```python
from build123d import *

# Parameters (mm, degrees)
BOSS_EXTRUDE1_DEPTH = 8
SKETCH4_R           = 2.6
CUT_EXTRUDE1_DEPTH  = 23
SKETCH5_R           = 1.5
CUT_EXTRUDE2_DEPTH  = 19.692452066


with BuildPart() as part:
    # Sketch1 → Boss-Extrude1 (new body)
    with BuildSketch(Plane(origin=(0, 0, 0), x_dir=(1, 0, 0), z_dir=(0, 1, 0))):
        with BuildLine():
            ThreePointArc((-2.619011045, 11.679969227), (-2.794341005, 11.639267947), (-2.969039138, 11.595934917))
            ThreePointArc((-2.969039138, 11.595934917), (-3.464080507, 10.661343548), (-4.413916411, 11.126465832))
            ThreePointArc((-4.413916411, 11.126465832), (-4.580720685, 11.058838004), (-4.746489215, 10.988709666))
            ThreePointArc((-4.746489215, 10.988709666), (-5.089233502, 9.988183136), (-6.100136506, 10.298991922))
            ThreePointArc((-6.100136506, 10.298991922), (-6.25430782, 10.206102767), (-6.407064974, 10.110905915))
            ThreePointArc((-6.407064974, 10.110905915), (-6.589072678, 9.069080507), (-7.636150994, 9.21792265))
            ThreePointArc((-7.636150994, 9.21792265), (-7.773893139, 9.102059408), (-7.909877531, 8.984138103))
            ThreePointArc((-7.909877531, 8.984138103), (-7.926667017, 7.926667017), (-8.984138103, 7.909877531))
            ThreePointArc((-8.984138103, 7.909877531), (-9.102059408, 7.773893139), (-9.21792265, 7.636150994))
            ThreePointArc((-9.21792265, 7.636150994), (-9.069080507, 6.589072678), (-10.110905915, 6.407064974))
            ThreePointArc((-10.110905915, 6.407064974), (-10.206102767, 6.25430782), (-10.298991922, 6.100136506))
            ThreePointArc((-10.298991922, 6.100136506), (-9.988183136, 5.089233502), (-10.988709666, 4.746489215))
            ThreePointArc((-10.988709666, 4.746489215), (-11.058838004, 4.580720685), (-11.126465832, 4.413916411))
            ThreePointArc((-11.126465832, 4.413916411), (-10.661343548, 3.464080507), (-11.595934917, 2.969039138))
            ThreePointArc((-11.595934917, 2.969039138), (-11.639267947, 2.794341005), (-11.679969227, 2.619011045))
            ThreePointArc((-11.679969227, 2.619011045), (-11.071986298, 1.753630353), (-11.917629765, 1.118481464))
            ThreePointArc((-11.917629765, 1.118481464), (-11.933100485, 0.939155376), (-11.945873016, 0.759616935))
            ThreePointArc((-11.945873016, 0.759616935), (-11.21, 0), (-11.945873016, -0.759616935))
            ThreePointArc((-11.945873016, -0.759616935), (-11.933100485, -0.939155376), (-11.917629765, -1.118481464))
            ThreePointArc((-11.917629765, -1.118481464), (-11.071986298, -1.753630353), (-11.679969227, -2.619011045))
            ThreePointArc((-11.679969227, -2.619011045), (-11.639267947, -2.794341005), (-11.595934917, -2.969039138))
            ThreePointArc((-11.595934917, -2.969039138), (-10.661343548, -3.464080507), (-11.126465832, -4.413916411))
            ThreePointArc((-11.126465832, -4.413916411), (-11.058838004, -4.580720685), (-10.988709666, -4.746489215))
            ThreePointArc((-10.988709666, -4.746489215), (-9.988183136, -5.089233502), (-10.298991922, -6.100136506))
            ThreePointArc((-10.298991922, -6.100136506), (-10.206102767, -6.25430782), (-10.110905915, -6.407064974))
            ThreePointArc((-10.110905915, -6.407064974), (-9.069080507, -6.589072678), (-9.21792265, -7.636150994))
            ThreePointArc((-9.21792265, -7.636150994), (-9.102059408, -7.773893139), (-8.984138103, -7.909877531))
            ThreePointArc((-8.984138103, -7.909877531), (-7.926667017, -7.926667017), (-7.909877531, -8.984138103))
            ThreePointArc((-7.909877531, -8.984138103), (-7.773893139, -9.102059408), (-7.636150994, -9.21792265))
            ThreePointArc((-7.636150994, -9.21792265), (-6.589072678, -9.069080507), (-6.407064974, -10.110905915))
            ThreePointArc((-6.407064974, -10.110905915), (-6.25430782, -10.206102767), (-6.100136506, -10.298991922))
            ThreePointArc((-6.100136506, -10.298991922), (-5.089233502, -9.988183136), (-4.746489215, -10.988709666))
            ThreePointArc((-4.746489215, -10.988709666), (-4.580720685, -11.058838004), (-4.413916411, -11.126465832))
            ThreePointArc((-4.413916411, -11.126465832), (-3.464080507, -10.661343548), (-2.969039138, -11.595934917))
            ThreePointArc((-2.969039138, -11.595934917), (-2.794341005, -11.639267947), (-2.619011045, -11.679969227))
            ThreePointArc((-2.619011045, -11.679969227), (-1.753630353, -11.071986298), (-1.118481464, -11.917629765))
            ThreePointArc((-1.118481464, -11.917629765), (-0.939155376, -11.933100485), (-0.759616935, -11.945873016))
            ThreePointArc((-0.759616935, -11.945873016), (0, -11.21), (0.759616935, -11.945873016))
            ThreePointArc((0.759616935, -11.945873016), (0.939155376, -11.933100485), (1.118481464, -11.917629765))
            ThreePointArc((1.118481464, -11.917629765), (1.753630353, -11.071986298), (2.619011045, -11.679969227))
            ThreePointArc((2.619011045, -11.679969227), (2.794341005, -11.639267947), (2.969039138, -11.595934917))
            ThreePointArc((2.969039138, -11.595934917), (3.464080507, -10.661343548), (4.413916411, -11.126465832))
            ThreePointArc((4.413916411, -11.126465832), (4.580720685, -11.058838004), (4.746489215, -10.988709666))
            ThreePointArc((4.746489215, -10.988709666), (5.089233502, -9.988183136), (6.100136506, -10.298991922))
            ThreePointArc((6.100136506, -10.298991922), (6.25430782, -10.206102767), (6.407064974, -10.110905915))
            ThreePointArc((6.407064974, -10.110905915), (6.589072678, -9.069080507), (7.636150994, -9.21792265))
            ThreePointArc((7.636150994, -9.21792265), (7.773893139, -9.102059408), (7.909877531, -8.984138103))
            ThreePointArc((7.909877531, -8.984138103), (7.926667017, -7.926667017), (8.984138103, -7.909877531))
            ThreePointArc((8.984138103, -7.909877531), (9.102059408, -7.773893139), (9.21792265, -7.636150994))
            ThreePointArc((9.21792265, -7.636150994), (9.069080507, -6.589072678), (10.110905915, -6.407064974))
            ThreePointArc((10.110905915, -6.407064974), (10.206102767, -6.25430782), (10.298991922, -6.100136506))
            ThreePointArc((10.298991922, -6.100136506), (9.988183136, -5.089233502), (10.988709666, -4.746489215))
            ThreePointArc((10.988709666, -4.746489215), (11.058838004, -4.580720685), (11.126465832, -4.413916411))
            ThreePointArc((11.126465832, -4.413916411), (10.661343548, -3.464080507), (11.595934917, -2.969039138))
            ThreePointArc((11.595934917, -2.969039138), (11.639267947, -2.794341005), (11.679969227, -2.619011045))
            ThreePointArc((11.679969227, -2.619011045), (11.071986298, -1.753630353), (11.917629765, -1.118481464))
            ThreePointArc((11.917629765, -1.118481464), (11.933100485, -0.939155376), (11.945873016, -0.759616935))
            ThreePointArc((11.945873016, -0.759616935), (11.21, 0), (11.945873016, 0.759616935))
            ThreePointArc((11.945873016, 0.759616935), (11.933100485, 0.939155376), (11.917629765, 1.118481464))
            ThreePointArc((11.917629765, 1.118481464), (11.071986298, 1.753630353), (11.679969227, 2.619011045))
            ThreePointArc((11.679969227, 2.619011045), (11.639267947, 2.794341005), (11.595934917, 2.969039138))
            ThreePointArc((11.595934917, 2.969039138), (10.661343548, 3.464080507), (11.126465832, 4.413916411))
            ThreePointArc((11.126465832, 4.413916411), (11.058838004, 4.580720685), (10.988709666, 4.746489215))
            ThreePointArc((10.988709666, 4.746489215), (9.988183136, 5.089233502), (10.298991922, 6.100136506))
            ThreePointArc((10.298991922, 6.100136506), (10.206102767, 6.25430782), (10.110905915, 6.407064974))
            ThreePointArc((10.110905915, 6.407064974), (9.069080507, 6.589072678), (9.21792265, 7.636150994))
            ThreePointArc((9.21792265, 7.636150994), (9.102059408, 7.773893139), (8.984138103, 7.909877531))
            ThreePointArc((8.984138103, 7.909877531), (7.926667017, 7.926667017), (7.909877531, 8.984138103))
            ThreePointArc((7.909877531, 8.984138103), (7.773893139, 9.102059408), (7.636150994, 9.21792265))
            ThreePointArc((7.636150994, 9.21792265), (6.589072678, 9.069080507), (6.407064974, 10.110905915))
            ThreePointArc((6.407064974, 10.110905915), (6.25430782, 10.206102767), (6.100136506, 10.298991922))
            ThreePointArc((6.100136506, 10.298991922), (5.089233502, 9.988183136), (4.746489215, 10.988709666))
            ThreePointArc((4.746489215, 10.988709666), (4.580720685, 11.058838004), (4.413916411, 11.126465832))
            ThreePointArc((4.413916411, 11.126465832), (3.464080507, 10.661343548), (2.969039138, 11.595934917))
            ThreePointArc((2.969039138, 11.595934917), (2.794341005, 11.639267947), (2.619011045, 11.679969227))
            ThreePointArc((2.619011045, 11.679969227), (1.753630353, 11.071986298), (1.118481464, 11.917629765))
            ThreePointArc((1.118481464, 11.917629765), (0.939155376, 11.933100485), (0.759616935, 11.945873016))
            ThreePointArc((0.759616935, 11.945873016), (0, 11.21), (-0.759616935, 11.945873016))
            ThreePointArc((-0.759616935, 11.945873016), (-0.939155376, 11.933100485), (-1.118481464, 11.917629765))
            ThreePointArc((-1.118481464, 11.917629765), (-1.753630353, 11.071986298), (-2.619011045, 11.679969227))
        make_face()
    extrude(amount=BOSS_EXTRUDE1_DEPTH)

    # Sketch4 → Cut-Extrude1 (cut)
    with BuildSketch(Plane.XZ):
        with Locations(Location((0, 0, 0), (0, 0, 270))):
            Circle(SKETCH4_R)
    extrude(amount=-CUT_EXTRUDE1_DEPTH, mode=Mode.SUBTRACT)

    # Sketch5 → Cut-Extrude2 (cut, through all)
    with BuildSketch(Plane.XZ):
        with Locations(Location((0, 7.5, 0), (0, 0, 270))):
            Circle(SKETCH5_R)
        with Locations(Location((7.5, 0, 0), (0, 0, 270))):
            Circle(SKETCH5_R)
        with Locations(Location((0, -7.5, 0), (0, 0, 270))):
            Circle(SKETCH5_R)
        with Locations(Location((-7.5, 0, 0), (0, 0, 270))):
            Circle(SKETCH5_R)
    extrude(amount=-CUT_EXTRUDE2_DEPTH, mode=Mode.SUBTRACT)


solid = part.part
```
Input: part model. Units: mm. Frame: model coordinates. Give positions to 0.01 mm unless a question says otherwise; leave off trailing zeros. Loops run counter-clockwise (first coordinate to the right, second up) from the corner with the lowest first, then second, coordinate; pieces in that order, holes last. Notation, with made-up numbers: (68.5, 83.5) -> (120.5, 83.5) arc R26 ccw to (120.5, 122.5) -> close; hole circle Ø4 at (64.25, -34). An arc over 180 degrees is marked (long way). Use a Markdown table: item, result.
Q1. Section query C-C, the plane y = 6.5. State how many separate pieces and enclosed holes the cut face has, plus the area to 3 significant figures.
Entries:
| item | result |
|---|---|
| separate pieces | 1 |
| enclosed holes | 5 |
| area | 365 mm² |
Q2. Section query A-A, the plane x = 0. Return the cut outline in (y, z), plus the area to 3 significant figures.
Entries:
| item | result |
|---|---|
| outline | (0, -11.21) -> (8, -11.21) -> (8, -9) -> (0, -9) -> close; (0, -6) -> (8, -6) -> (8, -2.6) -> (0, -2.6) -> close; (0, 2.6) -> (8, 2.6) -> (8, 6) -> (0, 6) -> close; (0, 9) -> (8, 9) -> (8, 11.21) -> (0, 11.21) -> close |
| area | 89.8 mm² |
Q3. Section query B-B, the plane z = 0. Return the cut outline in (x, y), plus the area to 3 significant figures.
Entries:
| item | result |
|---|---|
| outline | (-11.21, 0) -> (-9, 0) -> (-9, 8) -> (-11.21, 8) -> close; (-6, 0) -> (-2.6, 0) -> (-2.6, 8) -> (-6, 8) -> close; (2.6, 0) -> (6, 0) -> (6, 8) -> (2.6, 8) -> close; (9, 0) -> (11.21, 0) -> (11.21, 8) -> (9, 8) -> close |
| area | 89.8 mm² |
Q4. Pull-direction query (Z, two-part tool) for faces 1 (the cylindrical face through (-0.02, 3.94, 11.21)), 2 (the cylindrical face through (11.21, 3.94, 0.02)), 3 (the flat face through (0, 8, -3)); classes: pulls with the +Z half, pulls with the -Z half, needs draft (parallel to the pull), parting line crosses it, or undercut.
Entries:
| item | result |
|---|---|
| face 1 | pulls with the +Z half |
| face 2 | undercut |
| face 3 | needs draft |
Q5. Section query D-D, the plane z = 9.5. Return the cut outline in (x, y), plus the area to 3 significant figures.
Entries:
| item | result |
|---|---|
| outline | (-6.3, 0) -> (6.3, 0) -> (6.3, 8) -> (-6.3, 8) -> close |
| area | 101 mm² |
Q6. First-contact query: P1, Ø4, axis at y = 7, z = 8.5, coming from the +X side; P2, Ø1, axis at x = 9, y = 2.5, coming from the +Z side. Flat tips, straight axial feed; report the tip coordinate or a pass-through.
Entries:
| item | result |
|---|---|
| P1 | stops at x = 9.22 |
| P2 | stops at z = 7.91 |
Q7. Ray query, probe 1 along X at (y, z) = (2.5, 0); probe 2 along Z at (x, y) = (-1, 3); probe 3 along X at (y, z) = (6.75, 6.5). Return the intervals inside material, ascending. Write a range as from..to.
Entries:
| item | result |
|---|---|
| probe 1 | x = -11.21..-9, -6..-2.6, 2.6..6, 9..11.21 |
| probe 2 | z = -11.93..-8.62, -6.38..-2.4, 2.4..6.38, 8.62..11.93 |
| probe 3 | x = -9.14..-1.12, 1.12..9.14 |
